Model file for the job. Use its own axes, mm. A direction names the side the tool comes from. Give positions to 0.01 mm unless a question says otherwise; leave off trailing zeros. Write each loop counter-clockwise with the first axis right and the second up, starting at its lowest first coordinate (ties: lowest second). Pieces come first, ordered by that corner, then holes.
```python
from build123d import *

# Parameters (mm, degrees)
PAD004_DEPTH           = 153
PAD005_DEPTH           = 139
SKETCH007_W            = 124.6
SKETCH007_H            = 126
PAD006_DEPTH           = 3
POCKET002_DEPTH        = 124.601
LINEARPATTERN001_COUNT = 5
LINEARPATTERN001_PITCH = 22.5
POCKET003_DEPTH        = 4
LINEARPATTERN002_COUNT = 5
LINEARPATTERN002_PITCH = 22.5
SKETCH015_R            = 2
POCKET006_DEPTH        = 5
SKETCH016_W            = 12.436569
SKETCH016_H            = 17.864411
SKETCH016_W_2          = 20
SKETCH016_H_2          = 20
POCKET008_DEPTH        = 5
PAD007_DEPTH           = 3
PAD008_DEPTH           = 3


with BuildPart() as part:
    # Sketch006 → Pad004 (new body)
    with BuildSketch(Plane.XY):
        Polygon((62.3, 64.5), (-62.3, 64.5), (-62.3, -61.5), (-59.3, -61.5), (-59.3, 61.5), (59.3, 61.5), (59.3, -61.5), (62.3, -61.5), align=None)
    extrude(amount=PAD004_DEPTH)

    # Sketch008 (on DatumPlane) → Pad005 (join)
    with BuildSketch(Plane.XY.offset(153)):
        Polygon((-59.3, 59.5), (-57.299999, 61.5), (-59.3, 61.5), align=None)
    pad005 = extrude(amount=-PAD005_DEPTH)

    # Mirrored001: Pad005 across Sketch008 V_Axis
    add(pad005.mirror(Plane(origin=(0, 0, 153), x_dir=(0, 0, 1), z_dir=(1, 0, 0))))

    # Sketch007 (on DatumPlane) → Pad006 (join)
    with BuildSketch(Plane.XY.offset(153)):
        with Locations((0, 1.5)):
            Rectangle(SKETCH007_W, SKETCH007_H)
    extrude(amount=PAD006_DEPTH)

    # Sketch010 (on DatumPlane) → Pocket002 (cut, through all)
    with BuildSketch(Plane.YZ.offset(62.3)):
        with BuildLine():
            Line((-46, -89.527603), (-46, 133))
            ThreePointArc((-42, 133), (-44, 135), (-46, 133))
            Line((-42, 133), (-42, -89.527603))
            ThreePointArc((-46, -89.527603), (-44, -91.527603), (-42, -89.527603))
        make_face()
    pocket002 = extrude(amount=-POCKET002_DEPTH, mode=Mode.SUBTRACT)

    # LinearPattern001: Pocket002 ×5
    with Locations(*[(0, i * LINEARPATTERN001_PITCH, 0) for i in range(1, LINEARPATTERN001_COUNT)]):
        add(pocket002, mode=Mode.SUBTRACT)

    # Sketch011 (on Face13 of Pad006) → Pocket003 (cut)
    with BuildSketch(Plane.XY.offset(156)):
        with BuildLine():
            Line((-45.3, -42), (45.3, -42))
            ThreePointArc((45.3, -46), (47.3, -44), (45.3, -42))
            Line((45.3, -46), (-45.3, -46))
            ThreePointArc((-45.3, -42), (-47.3, -44), (-45.3, -46))
        make_face()
    pocket003 = extrude(amount=-POCKET003_DEPTH, mode=Mode.SUBTRACT)

    # LinearPattern002: Pocket003 ×5
    with Locations(*[(0, i * LINEARPATTERN002_PITCH, 0) for i in range(1, LINEARPATTERN002_COUNT)]):
        add(pocket003, mode=Mode.SUBTRACT)

    # Sketch015 (on DatumPlane) → Pocket006 (cut)
    with BuildSketch(Plane.XZ.offset(-64.5)):
        with Locations((-45.035357, 71.063824)):
            Circle(SKETCH015_R)
        with BuildLine():
            Line((-27.322272, 78.383734), (-27.322272, 133))
            ThreePointArc((-23.322272, 133), (-25.322272, 135), (-27.322272, 133))
            Line((-23.322272, 133), (-23.322272, 78.383734))
            ThreePointArc((-27.322272, 78.383734), (-25.322272, 76.383734), (-23.322272, 78.383734))
        make_face()
        with BuildLine():
            Line((-12.322272, 78.383734), (-12.322272, 133))
            ThreePointArc((-8.322272, 133), (-10.322272, 135), (-12.322272, 133))
            Line((-8.322272, 133), (-8.322272, 78.383734))
            ThreePointArc((-12.322272, 78.383734), (-10.322272, 76.383734), (-8.322272, 78.383734))
        make_face()
        with BuildLine():
            Line((2.677728, 78.383734), (2.677728, 133))
            ThreePointArc((6.677728, 133), (4.677728, 135), (2.677728, 133))
            Line((6.677728, 133), (6.677728, 78.383734))
            ThreePointArc((2.677728, 78.383734), (4.677728, 76.383734), (6.677728, 78.383734))
        make_face()
        with BuildLine():
            Line((-42.322272, 78.383734), (-42.322272, 133))
            ThreePointArc((-38.322272, 133), (-40.322272, 135), (-42.322272, 133))
            Line((-38.322272, 133), (-38.322272, 78.383734))
            ThreePointArc((-42.322272, 78.383734), (-40.322272, 76.383734), (-38.322272, 78.383734))
        make_face()
    extrude(amount=POCKET006_DEPTH, mode=Mode.SUBTRACT)

    # Sketch016 (on DatumPlane) → Pocket008 (cut)
    with BuildSketch(Plane.YZ.offset(62.3)):
        with Locations((41.675534, 17.748693)):
            Rectangle(SKETCH016_W, SKETCH016_H)
        with Locations((44.407095, 63.300186)):
            Rectangle(SKETCH016_W_2, SKETCH016_H_2)
        with Locations((44.279243, 130.745399)):
            Rectangle(SKETCH016_W_2, SKETCH016_H_2)
    extrude(amount=-POCKET008_DEPTH, mode=Mode.SUBTRACT)

    # Sketch017 (on DatumPlane) → Pad007 (join)
    with BuildSketch(Plane.YZ.offset(62.3)):
        Polygon((55.794507, 119.712103), (-56.964375, 30.887549), (-56.964375, 27.887549), (55.794507, 116.712103), align=None)
        Polygon((54.067337, 31.341833), (-55.976406, 119.712103), (-55.976406, 116.712103), (54.067337, 27.887549), align=None)
    extrude(amount=-PAD007_DEPTH)

    # Sketch018 (on DatumPlane) → Pad008 (join)
    with BuildSketch(Plane.YZ.offset(-62.3)):
        Polygon((55.794507, 119.712103), (-56.964375, 30.887549), (-56.964375, 27.887549), (55.794507, 116.712103), align=None)
        Polygon((54.067337, 31.341833), (-55.976406, 119.712103), (-55.976406, 116.712103), (54.067337, 27.887549), align=None)
    extrude(amount=PAD008_DEPTH)


with BuildPart() as part_1:
    # Body001 placement: moved
    add(part.part.moved(Location((1.4, 0, 110.1))))


solid = part_1.part
```
1. Pull direction X, two halves, no side cores. Call faces 3 (the flat face through (1, 61.5, 186)), 4 (the flat face through (1, 62, 110.1)), 5 (the flat face through (-60.9, -13, 187)), 6 (the flat face through (60.7, 1, 186)): +X half, -X half, draft (parallel to the pull), parting line (faces both ways), or undercut.
Calculated:
face 3: undercut
face 4: draft
face 5: -X half
face 6: undercut
2. Slice it at B-B, the plane y = 23.5. Write the cut outline in (x, z).
Calculated:
outline: (-60.9, 162.66) - (-57.9, 162.66) - (-57.9, 165.99) - (-60.9, 165.99) - close; (-60.9, 201.37) - (-57.9, 201.37) - (-57.9, 204.37) - (-60.9, 204.37) - close; (-60.9, 245.1) - (-57.9, 245.1) - (-57.9, 263.1) - (-45.9, 263.1) - (-45.9, 266.1) - (-60.9, 266.1) - close; (48.7, 263.1) - (60.7, 263.1) - (60.7, 245.1) - (63.7, 245.1) - (63.7, 266.1) - (48.7, 266.1) - close; (60.7, 162.66) - (63.7, 162.66) - (63.7, 165.99) - (60.7, 165.99) - close; (60.7, 201.37) - (63.7, 201.37) - (63.7, 204.37) - (60.7, 204.37) - close
3. Which spindle directions (+Z, -Z, +X, -X, +Y, -Y) get a long thin tool onto all of the face, cutting with end or side? Do faces 1 (the flat face through (1, -12, 266.1)), 2 (the flat face through (-57.9, 13, 186)). Say none if no direction does.
Calculated:
face 1: +Z, +X, -X, +Y, -Y
face 2: -Z, -Y
4. Pin check, flat tip, straight feed: P1, Ø2, axis at x = 48.5, z = 250, coming from the -Y side. Stop position of the tip, or through.
Calculated:
P1: stops at y = 61.5
5. Slice it at C-C, the plane y = 8. Write the cut outline in (x, z).
Calculated:
outline: (-60.9, 110.1) - (-57.9, 110.1) - (-57.9, 263.1) - (60.7, 263.1) - (60.7, 110.1) - (63.7, 110.1) - (63.7, 266.1) - (-60.9, 266.1) - close
6. Probe probe 1 along X at (y, z) = (43, 226); probe 2 along Z at (x, y) = (-34, -40); probe 3 along Y at (x, z) = (-46, 170). List the from-to ranges inside material, lowest first.
Calculated:
probe 1: x = -60.9 to -57.9, 60.7 to 63.7
probe 2: z = 263.1 to 266.1
probe 3: y = 61.5 to 64.5
7. Slice it at A-A, the plane x = -2.5. Write the cut outline in (y, z).
Calculated:
outline: (-61.5, 263.1) - (-46, 263.1) - (-46, 266.1) - (-61.5, 266.1) - close; (-42, 263.1) - (-23.5, 263.1) - (-23.5, 266.1) - (-42, 266.1) - close; (-19.5, 263.1) - (-1, 263.1) - (-1, 266.1) - (-19.5, 266.1) - close; (3, 263.1) - (21.5, 263.1) - (21.5, 266.1) - (3, 266.1) - close; (25.5, 263.1) - (44, 263.1) - (44, 266.1) - (25.5, 266.1) - close; (48, 263.1) - (61.5, 263.1) - (61.5, 110.1) - (64.5, 110.1) - (64.5, 266.1) - (48, 266.1) - close
8. Slice it at D-D, the plane z = 213. State how many separate pieces and enclosed holes the cut face has, and give its area (3 significant figures).
Calculated:
separate pieces: 15
enclosed holes: 0
area: 948 mm2
